```python
from build123d import *

# Parameters (mm, degrees)
SKETCH2_R           = 1
BOSS_EXTRUDE1_DEPTH = 3
FILLET1_R           = 1


with BuildPart() as part:
    # Sketch2 → Boss-Extrude1 (new body)
    with BuildSketch(Plane(origin=(0, 0, 0), x_dir=(1, 0, 0), z_dir=(0, 1, 0))):
        Polygon((20.748238747, 19.933341623), (14.748238747, 19.933341623), (14.748238747, 18.933341623), (11.748238747, 18.933341623), (11.748238747, 14.933341623), (14.748238747, 14.933341623), (14.748238747, 13.933341623), (15.43988716, 13.933341623), (17.267927311, -0.954850651), (23.22320422, -0.223634591), align=None)
        with Locations(Location((18.141595519, 16.546219938, 0), (0, 0, 270))):
            Circle(SKETCH2_R, mode=Mode.SUBTRACT)
        with Locations(Location((19.879957735, 2.388395834, 0), (0, 0, 270))):
            Circle(SKETCH2_R, mode=Mode.SUBTRACT)
    extrude(amount=BOSS_EXTRUDE1_DEPTH)

    # Fillet1
    fillet1_edges = [part.edges().sort_by_distance(p)[0] for p in [
        (20.748238747, 1.5, -19.933341623),
        (23.22320422, 1.5, 0.223634591),
        (17.267927311, 1.5, 0.954850651),
    ]]
    fillet(fillet1_edges, radius=FILLET1_R)


solid = part.part
```
Here's how the part is built. I have some questions about the finished solid (model axes, mm). A direction names the side the tool comes from. Coordinates: 2 decimals unless noted, no trailing zeros. Order: outer loops, then holes, each group sorted by start corner. A loop starts at its lowest first (then second) coordinate and runs counter-clockwise, first axis right, second up.
1) I need wall thicknesses on line 1 (Z direction, x = 14, y = 0.55); line 2 (Z direction, x = 17.75, y = 0.3); line 3 (Z direction, x = 20, y = 2.65). Which ranges of each line are inside material? Lowest first, please.
2) Imagine slicing it at B-B on y = 2.45. List the corners of the cut face in (x, z) for me, and give its area (3 significant figures).
3) Imagine slicing it at A-A on x = 18.5. List the corners of the cut face in (y, z) for me.
4) Imagine slicing it at C-C on x = 12.5. List the corners of the cut face in (y, z) for me.
5) Imagine slicing it at D-D on z = -18.25. List the corners of the cut face in (x, y) for me, and give its area (3 significant figures).
6) Will this pin go through, and if not, where does the flat tip stop? pin 1 (0.8 mm diameter, centred on y = 1, z = -14.5, fed in from -X).
7) We'd pull the mould along Z, two halves only. Please class faces 4 (the face through (17.165, 1.479, -16.763)), 5 (the face through (11.748, 1, -17)), 6 (the face through (17.532, 1.521, 0.635)), 7 (the face through (20.18, 1.479, -1.435)): +Z half, -Z half, draft (parallel to the pull), parting line (faces both ways), or undercut.
8) Which directions (+Z, -Z, +X, -X, +Y, -Y) give clear straight access to the entire face, cutting with the end or side of a thin tool? Please do faces 1 (the face through (14.748, 1.5, -19.4)), 2 (the face through (17, 1, -19.933)), 3 (the face through (14.748, 1.5, -14.4)).
Response values:
1. line 1: z = -18.93 to -14.93
1. line 2: z = -19.93 to -17.47, -15.63 to 0.76
1. line 3: z = -19.92 to -3.38, -1.4 to 0.62
2. outline: (11.75, -18.93) - (14.75, -18.93) - (14.75, -19.93) - (19.86, -19.93) arc R1 ccw to (20.86, -19.06) - (23.1, -0.77) arc R1 ccw to (22.23, 0.35) - (18.26, 0.83) arc R1 ccw to (17.15, -0.04) - (15.44, -13.93) - (14.75, -13.93) - (14.75, -14.93) - (11.75, -14.93) - close; hole circle Ø2 at (18.14, -16.55); hole circle Ø2 at (19.88, -2.39)
2. area: 131 mm2
3. outline: (0, -19.93) - (3, -19.93) - (3, -17.48) - (0, -17.48) - close; (0, -15.61) - (3, -15.61) - (3, 0.8) - (0, 0.8) - close
4. outline: (0, -18.93) - (3, -18.93) - (3, -14.93) - (0, -14.93) - close
5. outline: (11.75, 0) - (20.95, 0) - (20.95, 3) - (11.75, 3) - close
5. area: 27.6 mm2
6. pin 1: stops at x = 14.75
7. face 4: undercut
7. face 5: draft
7. face 6: +Z half
7. face 7: undercut
8. face 1: -Z, -X, +Y, -Y
8. face 2: -Z, +X, -X, +Y, -Y
8. face 3: +Z, -X, +Y, -Y
